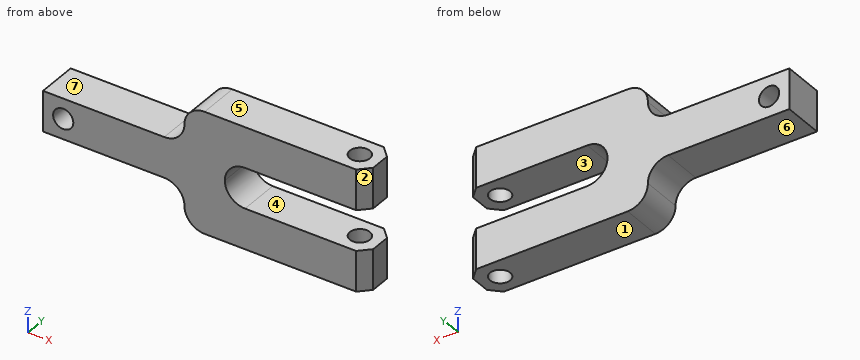
```python
from build123d import *

# Parameters (mm, degrees)
F0_R     = 6.35
F2_DEPTH = 25.4
F3_SIZE2 = 6.35
F3_SIZE  = 6.35
F1_R     = 6.35
F4_DEPTH = 127


with BuildPart() as f2:
    # F0 (on Front) → F2 (new body)
    with BuildSketch(Plane.XZ):
        with BuildLine():
            Line((0, 25.4), (0, 0))
            Line((0, 0), (76.2, 0))
            ThreePointArc((76.2, 0), (85.180256, -3.719744), (88.9, -12.7))
            ThreePointArc((88.9, -12.7), (92.619744, -21.680256), (101.6, -25.4))
            Line((101.6, -25.4), (203.2, -25.4))
            Line((203.2, -25.4), (203.2, 0))
            Line((203.2, 0), (127, 0))
            ThreePointArc((127, 0), (118.019744, 3.719744), (114.3, 12.7))
            ThreePointArc((114.3, 12.7), (118.019744, 21.680256), (127, 25.4))
            Line((127, 25.4), (203.2, 25.4))
            Line((203.2, 25.4), (203.2, 50.8))
            Line((203.2, 50.8), (101.6, 50.8))
            ThreePointArc((101.6, 50.8), (92.619744, 47.080256), (88.9, 38.1))
            ThreePointArc((88.9, 38.1), (85.180256, 29.119744), (76.2, 25.4))
            Line((76.2, 25.4), (0, 25.4))
        make_face()
        with Locations((12.7, 12.7)):
            Circle(F0_R, mode=Mode.SUBTRACT)
    extrude(amount=F2_DEPTH)

    # F3
    f3_edges = [f2.edges().sort_by_distance(p)[0] for p in [
        (203.2, -25.4, 38.1),
        (203.2, -25.4, -12.7),
        (203.2, 0, -12.7),
        (203.2, 0, 38.1),
    ]]
    chamfer(f3_edges, length=F3_SIZE, length2=F3_SIZE2)

    # F1 (on Top) → F4 (cut, symmetric)
    with BuildSketch(Plane.XY):
        with Locations((190.5, -12.7)):
            Circle(F1_R)
    extrude(amount=F4_DEPTH, both=True, mode=Mode.SUBTRACT)


solid = f2.part
```
CAD build for the part. Positions are in the model's coordinates, mm. Face numbers are marked on the shaded views. A direction names the side the tool comes from. Round coordinates to 2 decimals unless told otherwise and drop trailing zeros. Write each loop counter-clockwise with the first axis right and the second up, starting at its lowest first coordinate (ties: lowest second). Pieces come first, ordered by that corner, then holes. Notation, with made-up numbers: M -1,-25.75 L 10,-25.75 A20 ccw 10,-1.75 Z; hole C 45,51.5 d9. An arc over 180 degrees is marked long. One line per question, with ' | ' between items.
1. Probe L1, parallel to Z at x = 134, y = -10.25; L2, parallel to X at y = -11.75, z = 13; L3, parallel to Z at x = 12.7, y = -6.75. List the from-to ranges inside material, lowest first. Write a range as from..to.
Working result:
L1: -25.4..0, 25.4..50.8 | L2: 0..6.36, 19.04..114.3 | L3: 0..6.35, 19.05..25.4
2. Which spindle directions (+Z, -Z, +X, -X, +Y, -Y) get a long thin tool onto all of the face, cutting with end or side? Do the marked faces 5, 6 and 7. Say none if no direction does.
Working result:
face 5: +Z, +X, -X, +Y, -Y | face 6: -Z, -X, +Y, -Y | face 7: +Z, -X, +Y, -Y
3. Cut at C-C on y = -21. Write the cut outline in (x, z), and give its area (3 significant figures).
Working result:
outline: M 0,0 L 76.2,0 A12.7 cw 88.9,-12.7 A12.7 ccw 101.6,-25.4 L 201.25,-25.4 L 201.25,0 L 127,0 A12.7 cw 127,25.4 L 201.25,25.4 L 201.25,50.8 L 101.6,50.8 A12.7 ccw 88.9,38.1 A12.7 cw 76.2,25.4 L 0,25.4 Z; hole C 12.7,12.7 d12.7 | area: 8,550 mm2
4. Cut at D-D on x = 12.7. Write the cut outline in (y, z), and give its area (3 significant figures).
Working result:
outline: M -25.4,0 L 0,0 L 0,6.35 L -25.4,6.35 Z; M -25.4,19.05 L 0,19.05 L 0,25.4 L -25.4,25.4 Z | area: 323 mm2
5. Cut at A-A on y = -12.7. Write the cut outline in (x, z).
Working result:
outline: M 0,0 L 76.2,0 A12.7 cw 88.9,-12.7 A12.7 ccw 101.6,-25.4 L 184.15,-25.4 L 184.15,0 L 127,0 A12.7 cw 127,25.4 L 184.15,25.4 L 184.15,50.8 L 101.6,50.8 A12.7 ccw 88.9,38.1 A12.7 cw 76.2,25.4 L 0,25.4 Z; M 196.85,-25.4 L 203.2,-25.4 L 203.2,0 L 196.85,0 Z; M 196.85,25.4 L 203.2,25.4 L 203.2,50.8 L 196.85,50.8 Z; hole C 12.7,12.7 d12.7
6. Pin check, flat tips, straight feed: pin 1 Ø1 at (y, z) = (-19.5, 14.5) entering from +X; pin 2 Ø2 at (y, z) = (-21, 27.5) entering from -X; pin 3 Ø12.5 at (x, y) = (51.5, -17) entering from +Z. Stop position of each tip, or through.
Working result:
pin 1: x = 114.51 | pin 2: x = 81.37 | pin 3: z = 25.4
7. Mould opens along Z. For the marked faces 1, 2, 3 and 4 say: pulls with the +Z half, pulls with the -Z half, needs draft (parallel to the pull), parting line crosses it, or undercut.
Working result:
face 1: pulls with the -Z half | face 2: needs draft | face 3: undercut | face 4: undercut
8. Cut at B-B on x = 190.5. Write the cut outline in (y, z), and give its area (3 significant figures).
Working result:
outline: M -25.4,-25.4 L -19.05,-25.4 L -19.05,0 L -25.4,0 Z; M -25.4,25.4 L -19.05,25.4 L -19.05,50.8 L -25.4,50.8 Z; M -6.35,-25.4 L 0,-25.4 L 0,0 L -6.35,0 Z; M -6.35,25.4 L 0,25.4 L 0,50.8 L -6.35,50.8 Z | area: 645 mm2
